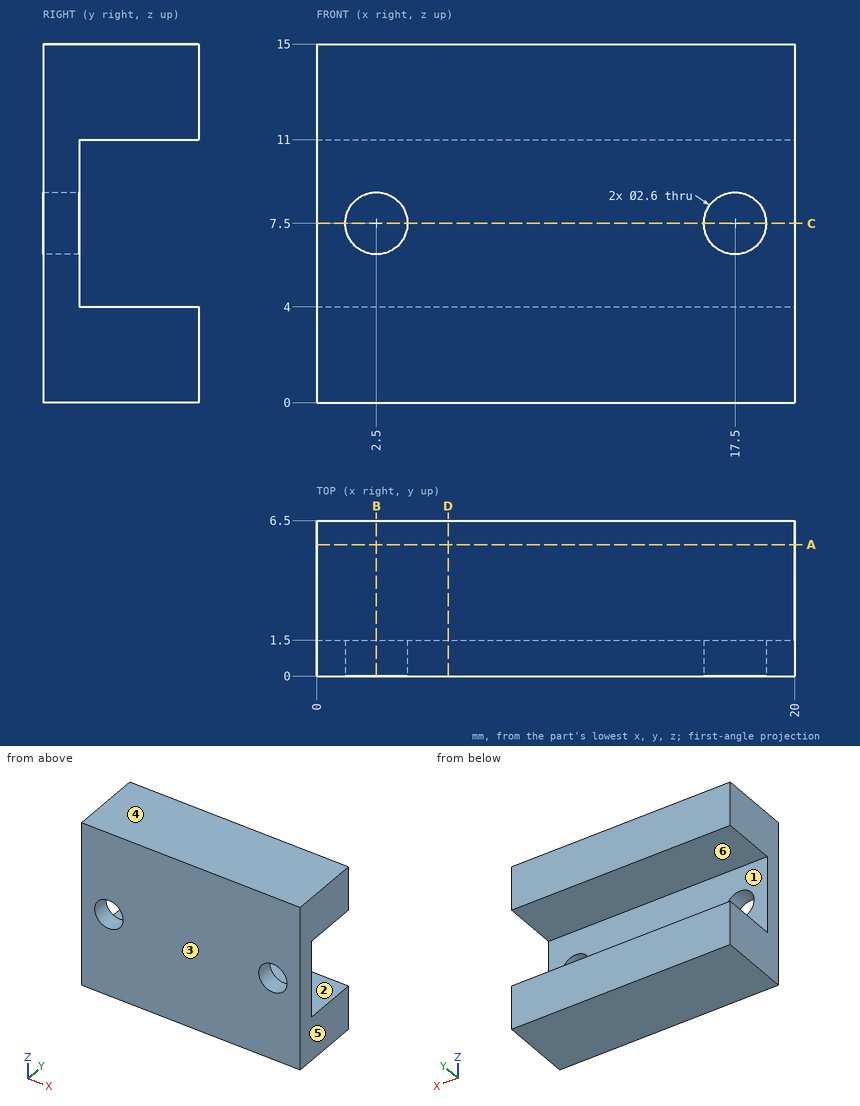
Job drawing, mm, ordinate dimensions from the low corner. One solid piece. A direction names the side the tool comes from. Coordinates: 2 decimals unless noted, no trailing zeros. Order: outer loops, then holes, each group sorted by start corner. A loop starts at its lowest first (then second) coordinate and runs counter-clockwise, first axis right, second up. Notation, with made-up numbers: (60.5, -10.5) - (75.5, -10.5) arc R19 ccw to (75.5, 15.5) - close; hole circle Ø10 at (34, 18.25). An arc over 180 degrees is marked (long way). Return JSON: item names as keys, results as strings. Group by question number.
1) Saw through at D-D, the plane x = 5.5. Write the cut outline in (y, z), plus the area to 3 significant figures.
2) Mould opens along Z. For the marked faces 1, 2, 3 and 4 say: released by +Z, released by -Z, zero draft, split by the parting line, or undercut.
3) Flat gauge pin, fed straight in: P1, Ø2, axis at x = 2.5, z = 7.5, coming from the -Y side. Where does the tip first touch, or does it go through?
4) Saw through at C-C, the plane z = 7.5. Write the cut outline in (x, y), plus the area to 3 significant figures.
5) Saw through at B-B, the plane x = 2.5. Write the cut outline in (y, z).
6) Tool access for the marked faces 5 and 6: list every direction of +Z, -Z, +X, -X, +Y, -Y with a clear straight run to the whole face (end or side of a thin tool).
7) Probe line 1 (X direction, y = 1.15, z = 7.5); line 2 (Z direction, x = 6.75, y = 6); line 3 (Y direction, x = 7.25, z = 6.5). List the from-to ranges inside material, lowest first. Write a range as from..to.
8) Saw through at A-A, the plane y = 5.5. Write the cut outline in (x, z).
Values found:
{
 "1": {"outline": "(0, 0) - (6.5, 0) - (6.5, 4) - (1.5, 4) - (1.5, 11) - (6.5, 11) - (6.5, 15) - (0, 15) - close", "area": "62.5 mm²"},
 "2": {"face 1": "undercut", "face 2": "undercut", "face 3": "zero draft", "face 4": "released by +Z"},
 "3": {"P1": "passes through"},
 "4": {"outline": "(0, 0) - (1.2, 0) - (1.2, 1.5) - (0, 1.5) - close; (3.8, 0) - (16.2, 0) - (16.2, 1.5) - (3.8, 1.5) - close; (18.8, 0) - (20, 0) - (20, 1.5) - (18.8, 1.5) - close", "area": "22.2 mm²"},
 "5": {"outline": "(0, 0) - (6.5, 0) - (6.5, 4) - (1.5, 4) - (1.5, 6.2) - (0, 6.2) - close; (0, 8.8) - (1.5, 8.8) - (1.5, 11) - (6.5, 11) - (6.5, 15) - (0, 15) - close"},
 "6": {"face 5": "+Z, -Z, +X, +Y, -Y", "face 6": "+X, -X, +Y"},
 "7": {"line 1": "x = 0..1.2, 3.8..16.2, 18.8..20", "line 2": "z = 0..4, 11..15", "line 3": "y = 0..1.5"},
 "8": {"outline": "(0, 0) - (20, 0) - (20, 4) - (0, 4) - close; (0, 11) - (20, 11) - (20, 15) - (0, 15) - close"}
}
